```python
from build123d import *

# Parameters (mm, degrees)
BOSS_EXTRUDE1_DEPTH = 100
CHAMFER1_SIZE       = 0.254


with BuildPart() as part:
    # Sketch1 → Boss-Extrude1 (new body)
    with BuildSketch(Plane.XY.offset(100)):
        with BuildLine():
            Line((1.658312395, 2.5), (-1.658312395, 2.5))
            ThreePointArc((-1.658312395, 2.5), (0, -3), (1.658312395, 2.5))
        make_face()
    extrude(amount=-BOSS_EXTRUDE1_DEPTH)

    # Chamfer1
    chamfer1_edges = [part.edges().sort_by_distance(p)[0] for p in [
        (0, 2.5, 100),
        (0, -3, 100),
        (0, -3, 0),
        (0, 2.5, 0),
    ]]
    chamfer(chamfer1_edges, length=CHAMFER1_SIZE)


solid = part.part
```
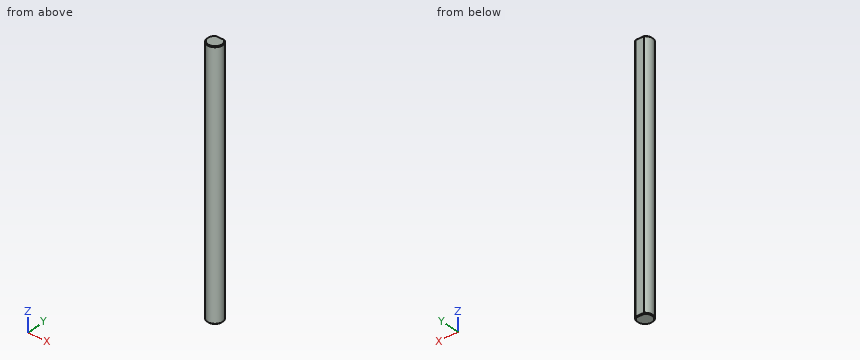
Read the model definition and answer for the solid it produces. Units are mm, in the model's axes. Coordinates: 2 decimals unless noted, no trailing zeros. Write each loop counter-clockwise with the first axis right and the second up, starting at its lowest first coordinate (ties: lowest second). Pieces come first, ordered by that corner, then holes. Notation, with made-up numbers: (28, 89) - (51, 89) arc R18 cw to (51, 119) - close; hole circle Ø10 at (77.25, 33). An arc over 180 degrees is marked (long way). Answer as a JSON object with one key per item and string values. Group by question number.
1. A cutting plane is placed at A-A (z = 46). Determine the outline of the cut face in (x, y), plus the area to 3 significant figures.
2. This flat-tipped pin is pushed along its axis until it touches: P1, Ø1, axis at y = 1, z = 84.5, coming from the +X side. Where does it stop, or does it pass through?
3. Consider L1, parallel to X at y = 0.3, z = 87; L2, parallel to X at y = -2.15, z = 83; L3, parallel to Y at x = -2, z = 72. Determine where each line is inside the solid, lowest interval first. Write a range as [from, to].
Worked out:
{
 "1": {"outline": "(-1.66, 2.5) arc R3 ccw (long way) to (1.66, 2.5) - close", "area": "27.1 mm²"},
 "2": {"P1": "stops at x = 2.96"},
 "3": {"L1": "x = [-2.98, 2.98]", "L2": "x = [-2.09, 2.09]", "L3": "y = [-2.24, 2.24]"}
}
